For this review, use the dimensioned drawing (mm, ordinates from the lowest corner) and the shaded views. A direction names the side the tool comes from. Coordinates: 2 decimals unless noted, no trailing zeros. Loops run counter-clockwise (first coordinate to the right, second up) from the corner with the lowest first, then second, coordinate; pieces in that order, holes last. Notation, with made-up numbers: M -14.5,5.5 L 4.5,5.5 A12 cw 4.5,22.5 Z; hole C -23,23 d4. An arc over 180 degrees is marked long. One line per item, written item: value.
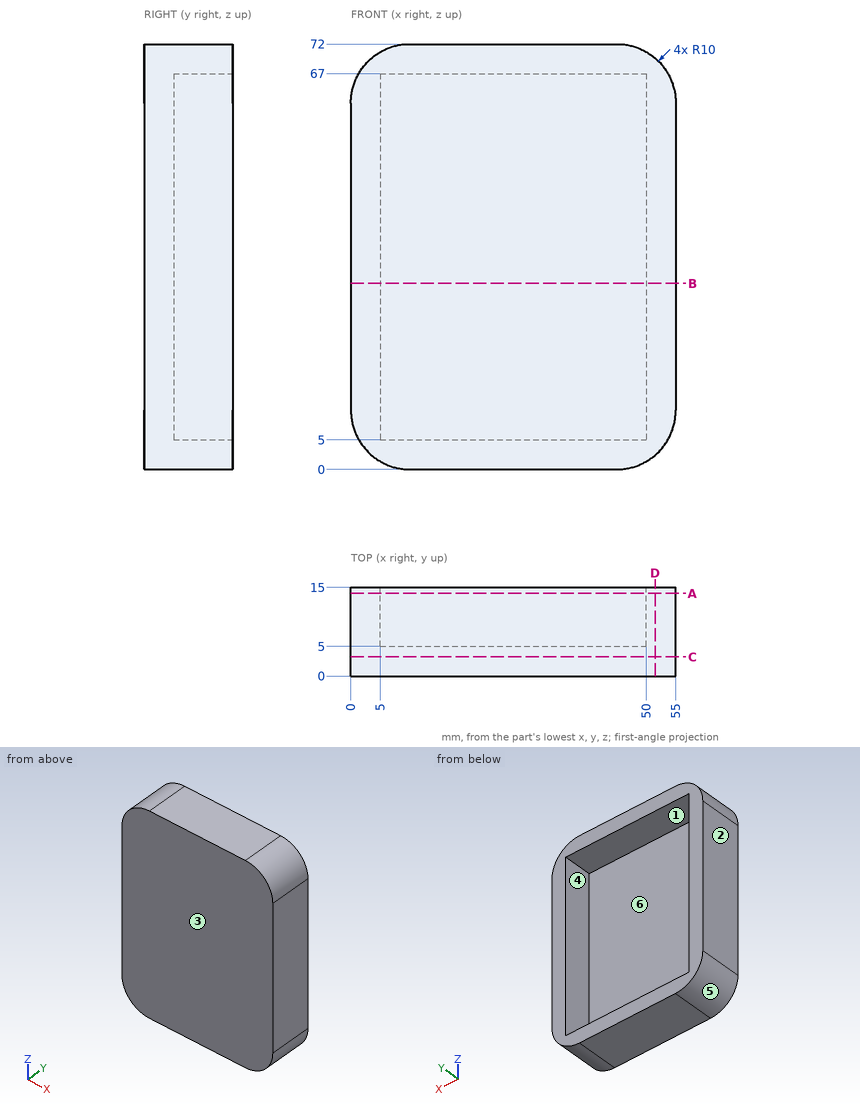
(1) Insertion check: pin 1 (22.5 mm diameter, centred on x = 33.5, z = 42.5, fed in from +Y). The pin has a flat end and moves straight along its axis. Give the tip position at first contact, or say it passes through.
Reply:
pin 1: stops at y = 5
(2) Tool access review of the marked faces 1 and 2: name each direction out of +Z, -Z, +X, -X, +Y, -Y from which nothing blocks a thin tool from reaching the whole face with its end or side.
Reply:
face 1: +Y
face 2: +Z, -Z, -X, +Y, -Y
(3) We need section C-C on y = 3.25. State the section outline as (x, z) points, then the cut area to 3 significant figures.
Reply:
outline: M 0,10 A10 ccw 10,0 L 45,0 A10 ccw 55,10 L 55,62 A10 ccw 45,72 L 10,72 A10 ccw 0,62 Z
area: 3,870 mm2
(4) We need section B-B on z = 31.5. State the section outline as (x, y) points.
Reply:
outline: M 0,0 L 55,0 L 55,15 L 50,15 L 50,5 L 5,5 L 5,15 L 0,15 Z
(5) Mouldability with a two-part tool opening along Z and no side actions: class the marked faces 3, 4, 5 and 6 as released by +Z, released by -Z, zero draft, split by the parting line, or undercut.
Reply:
face 3: zero draft
face 4: undercut
face 5: released by -Z
face 6: undercut
(6) We need section D-D on x = 51.5. State the section outline as (y, z) points.
Reply:
outline: M 0,2.4 L 15,2.4 L 15,69.6 L 0,69.6 Z
(7) We need section A-A on y = 14. State the section outline as (x, z) points, then the cut area to 3 significant figures.
Reply:
outline: M 0,10 A10 ccw 10,0 L 45,0 A10 ccw 55,10 L 55,62 A10 ccw 45,72 L 10,72 A10 ccw 0,62 Z; hole M 5,5 L 50,5 L 50,67 L 5,67 Z
area: 1,080 mm2
(8) To check wall thickness, follow line 1 along X through (y, z) = (10.25, 59); line 2 along Z through (x, y) = (14.5, 11.5); line 3 along Y through (x, z) = (29, 27.5). State the ranges of each line that lie inside material, in increasing order. Write a range as [from, to].
Reply:
line 1: x = [0, 5], [50, 55]
line 2: z = [0, 5], [67, 72]
line 3: y = [0, 5]
